```python
from build123d import *

# Parameters (mm, degrees)
BOSS_EXTRUDE1_DEPTH = 5


with BuildPart() as part:
    # Sketch1 → Boss-Extrude1 (new body)
    with BuildSketch(Plane(origin=(0, 0, 0), x_dir=(0, 0, -1), z_dir=(1, 0, 0))):
        with BuildLine():
            Line((-110, -6), (-90, -6))
            Line((-90, -6), (-90, 0))
            Line((-90, 0), (90, 0))
            Line((90, 0), (90, -6))
            Line((90, -6), (110, -6))
            Line((110, -6), (110, 94))
            Line((110, 94), (82.504621365, 89.151822902))
            Line((82.504621365, 89.151822902), (83.893806786, 81.273360878))
            Line((83.893806786, 81.273360878), (72.07611375, 79.189582746))
            Line((72.07611375, 79.189582746), (71.207872862, 84.113621511))
            Line((71.207872862, 84.113621511), (75.147103874, 84.808214222))
            Line((75.147103874, 84.808214222), (74.626159341, 87.762637481))
            Line((74.626159341, 87.762637481), (48.03635001, 83.074136684))
            Line((48.03635001, 83.074136684), (49.425535431, 75.195674659))
            Line((49.425535431, 75.195674659), (37.607842395, 73.111896527))
            Line((37.607842395, 73.111896527), (36.739601507, 78.035935292))
            Line((36.739601507, 78.035935292), (40.678832519, 78.730528003))
            Line((40.678832519, 78.730528003), (40.157887986, 81.684951262))
            Line((40.157887986, 81.684951262), (13.568078654, 76.996450465))
            Line((13.568078654, 76.996450465), (14.957264076, 69.117988441))
            Line((14.957264076, 69.117988441), (3.139571039, 67.034210309))
            Line((3.139571039, 67.034210309), (2.271330151, 71.958249074))
            Line((2.271330151, 71.958249074), (6.210561163, 72.652841785))
            Line((6.210561163, 72.652841785), (5.68961663, 75.607265044))
            Line((5.68961663, 75.607265044), (-20.900192701, 70.918764247))
            Line((-20.900192701, 70.918764247), (-19.51100728, 63.040302223))
            Line((-19.51100728, 63.040302223), (-31.328700316, 60.956524091))
            Line((-31.328700316, 60.956524091), (-32.196941204, 65.880562856))
            Line((-32.196941204, 65.880562856), (-28.257710192, 66.575155566))
            Line((-28.257710192, 66.575155566), (-28.778654725, 69.529578826))
            Line((-28.778654725, 69.529578826), (-55.368464057, 64.841078029))
            Line((-55.368464057, 64.841078029), (-53.979278635, 56.962616004))
            Line((-53.979278635, 56.962616004), (-65.796971671, 54.878837872))
            Line((-65.796971671, 54.878837872), (-66.66521256, 59.802876637))
            Line((-66.66521256, 59.802876637), (-62.725981548, 60.497469348))
            Line((-62.725981548, 60.497469348), (-63.246926081, 63.451892607))
            Line((-63.246926081, 63.451892607), (-77.735825896, 60.897108649))
            ThreePointArc((-77.735825896, 60.897108649), (-98.082925814, 50.934591362), (-110, 31.66701319))
            Line((-110, 31.66701319), (-110, 24.130960335))
            Line((-110, 24.130960335), (-102, 24.130960335))
            Line((-102, 24.130960335), (-102, 12.130960335))
            Line((-102, 12.130960335), (-106.999710258, 12.07713347))
            Line((-106.999710258, 12.07713347), (-107.000482929, 16.077133396))
            Line((-107.000482929, 16.077133396), (-110, 16.130960335))
            Line((-110, 16.130960335), (-110, -6))
        make_face()
    extrude(amount=BOSS_EXTRUDE1_DEPTH)


solid = part.part
```
Work out the finished part from the listing and answer in its coordinate system (mm). A direction names the side the tool comes from. Coordinates: 2 decimals unless noted, no trailing zeros. Order: outer loops, then holes, each group sorted by start corner. A loop starts at its lowest first (then second) coordinate and runs counter-clockwise, first axis right, second up. Notation, with made-up numbers: M -1.75,20 L 40.25,20 A24 cw 40.25,43 Z; hole C 23,-34 d8. An arc over 180 degrees is marked long. Use CSV: the item, a comma, the result in double quotes.
1) Determine the mould class of faces 4 (the face through (2, -3, -90)), 5 (the face through (2.46, 68.09, -9.13)), 6 (the face through (2.465, 62.192, 70.39)) for opening direction Y: released by +Y, released by -Y, zero draft, split by the parting line, or undercut.
Worked out:
face 4,"zero draft"
face 5,"undercut"
face 6,"released by +Y"
2) Consider line 1 (Y direction, x = 0.35, z = -23.5); line 2 (Y direction, x = 1, z = 11); line 3 (Z direction, x = 1.2, y = 89). Determine where each line is inside the solid, lowest interval first. Write a range as [from, to].
Worked out:
line 1,"y = [0, 78.75]"
line 2,"y = [0, 72.66]"
line 3,"z = [-110, -82.53]"
3) Section A-A on y = 20.5 is taken. Write down the section's boundary in (x, z), plus the area to 3 significant figures.
Worked out:
outline,"M 0,-110 L 5,-110 L 5,102 L 0,102 Z"
area,"1,060 mm^2"
4) Flat-ended cylindrical pins translate along their axes: pin 1 Ø1.5 at (x, z) = (4.5, 21) entering from +Y; pin 2 Ø1.5 at (x, y) = (3, 20) entering from +Z; pin 3 Ø1.5 at (x, z) = (1.5, 33.5) entering from -Y. Find the tip coordinate at first contact, or state that the pin passes through.
Worked out:
pin 1,"stops at y = 71.03"
pin 2,"stops at z = 102"
pin 3,"stops at y = 0"
5) Section B-B on z = 49 is taken. Write down the section's boundary in (x, y).
Worked out:
outline,"M 0,0 L 5,0 L 5,65.96 L 0,65.96 Z"
6) For faces 1 (the face through (2, -3, 90)), 2 (the face through (2, 5, 110)), 3 (the face through (2.465, 62.013, 25.337)), determine the directions among +Z, -Z, +X, -X, +Y, -Y from which every point of the face is accessible in a straight line to the end or side of a thin tool.
Worked out:
face 1,"+X, -X, -Y"
face 2,"+Z, +X, -X, +Y, -Y"
face 3,"+X, -X"
